```python
from build123d import *

# Parameters (mm, degrees)
SKETCH1_W           = 42
SKETCH1_H           = 66
BOSS_EXTRUDE1_DEPTH = 5
D_GAGEMENT_M51_D    = 5.5
CUT_EXTRUDE1_DEPTH  = 40.433488306


with BuildPart() as part:
    # Sketch1 → Boss-Extrude1 (new body)
    with BuildSketch(Plane.XY):
        Rectangle(SKETCH1_W, SKETCH1_H)
    extrude(amount=BOSS_EXTRUDE1_DEPTH)

    # Dégagement M51 (through all)
    with Locations(Plane.XY.offset(5)):
        with Locations((11, 18), (-11, 18), (0, -23)):
            Hole(D_GAGEMENT_M51_D / 2)

    # Sketch5 → Cut-Extrude1 (cut, through all)
    with BuildSketch(Plane.XY.offset(5)):
        with BuildLine():
            Line((-13.75, 13), (-13.75, 23))
            ThreePointArc((-13.75, 23), (-11, 25.75), (-8.25, 23))
            Line((-8.25, 23), (-8.25, 13))
            ThreePointArc((-8.25, 13), (-11, 10.25), (-13.75, 13))
        make_face()
        with BuildLine():
            Line((8.25, 13), (8.25, 23))
            ThreePointArc((8.25, 23), (11, 25.75), (13.75, 23))
            Line((13.75, 23), (13.75, 13))
            ThreePointArc((13.75, 13), (11, 10.25), (8.25, 13))
        make_face()
    extrude(amount=-CUT_EXTRUDE1_DEPTH, mode=Mode.SUBTRACT)


solid = part.part
```
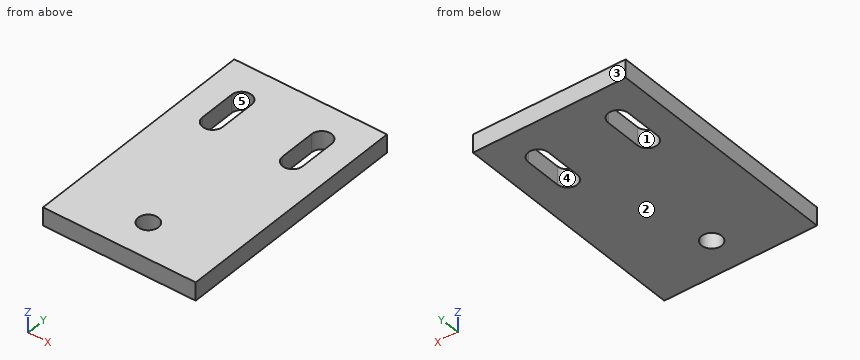
Verification items for the finished model (mm, model axes). Face numbers are marked on the shaded views. A direction names the side the tool comes from. Coordinates: 2 decimals unless noted, no trailing zeros. Write each loop counter-clockwise with the first axis right and the second up, starting at its lowest first coordinate (ties: lowest second). Pieces come first, ordered by that corner, then holes. Notation, with made-up numbers: M -30,22 L -26,22 A18 ccw -26,35 Z; hole C 23,-7.5 d8. An arc over 180 degrees is marked long. Answer as a JSON object with one key per item and string values. Group by question number.
(1) Gauge pin test, flat end, axial feed: pin 1 (3.5 mm diameter, centred on x = 0, y = -23, fed in from +Z). Record the tip position at first contact, or that the pin passes through.
(2) Release check for a two-part mould opening along X. For the marked faces 3, 4 and 5 record: +X half, -X half, draft (parallel to the pull), parting line (faces both ways), or undercut.
(3) Tool access check on the marked faces 1 and 2. Record the directions out of +Z, -Z, +X, -X, +Y, -Y that give a thin tool (end or side, any length) a straight path to the whole face; none if there is none.
(4) Cross-section at C-C, the plane z = 2.05. Record the cut outline in (x, y), and give its area (3 significant figures).
(5) Cross-section at A-A, the plane y = 18. Record the cut outline in (x, z), and give its area (3 significant figures).
(6) Material ranges on line 1 (X direction, y = 13, z = 0.7); line 2 (Y direction, x = 0, z = 1.7); line 3 (X direction, y = 11.5, z = 4.7), recorded low to high.
(7) Cross-section at D-D, the plane y = -23. Record the cut outline in (x, z), and give its area (4 significant figures).
(8) Cross-section at B-B, the plane x = 11. Record the cut outline in (y, z), and give its area (4 significant figures).
Reply:
{
 "1": {"pin 1": "through"},
 "2": {"face 3": "draft", "face 4": "undercut", "face 5": "undercut"},
 "3": {"face 1": "+Z, -Z", "face 2": "-Z, +X, -X, +Y, -Y"},
 "4": {"outline": "M -21,-33 L 21,-33 L 21,33 L -21,33 Z; hole M -13.75,13 A2.75 ccw -8.25,13 L -8.25,23 A2.75 ccw -13.75,23 Z; hole C 0,-23 d5.5; hole M 8.25,13 A2.75 ccw 13.75,13 L 13.75,23 A2.75 ccw 8.25,23 Z", "area": "2,590 mm²"},
 "5": {"outline": "M -21,0 L -13.75,0 L -13.75,5 L -21,5 Z; M -8.25,0 L 8.25,0 L 8.25,5 L -8.25,5 Z; M 13.75,0 L 21,0 L 21,5 L 13.75,5 Z", "area": "155 mm²"},
 "6": {"line 1": "-21 to -13.75, -8.25 to 8.25, 13.75 to 21", "line 2": "-33 to -25.75, -20.25 to 33", "line 3": "-21 to -13.3, -8.7 to 8.7, 13.3 to 21"},
 "7": {"outline": "M -21,0 L -2.75,0 L -2.75,5 L -21,5 Z; M 2.75,0 L 21,0 L 21,5 L 2.75,5 Z", "area": "182.5 mm²"},
 "8": {"outline": "M -33,0 L 10.25,0 L 10.25,5 L -33,5 Z; M 25.75,0 L 33,0 L 33,5 L 25.75,5 Z", "area": "252.5 mm²"}
}
